```python
from build123d import *

# Parameters (mm, degrees)
SKETCH2_W                  = 68
SKETCH2_H                  = 65
BOSS_EXTRUDE1_DEPTH        = 3
SKETCH3_W                  = 3
SKETCH3_H                  = 65
BOSS_EXTRUDE2_DEPTH        = 62
CUT_EXTRUDE1_DEPTH         = 78.821912081
SKETCH5_R                  = 19.05
CUT_EXTRUDE2_DEPTH         = 100.525122457
F_5_5_5_5_DIAMETER_HOLE1_D = 5.5
CHAMFER1_SIZE              = 5
CHAMFER2_SIZE              = 5
CHAMFER3_SIZE              = 5
BOSS_EXTRUDE3_DEPTH        = 2.5
BOSS_EXTRUDE4_DEPTH        = 2.5


with BuildPart() as part:
    # Sketch2 → Boss-Extrude1 (new body)
    with BuildSketch(Plane(origin=(0, 0, 0), x_dir=(1, 0, 0), z_dir=(0, 1, 0))):
        Rectangle(SKETCH2_W, SKETCH2_H)
    extrude(amount=BOSS_EXTRUDE1_DEPTH)

    # Sketch3 → Boss-Extrude2 (add)
    with BuildSketch(Plane(origin=(0, 3, 0), x_dir=(1, 0, 0), z_dir=(0, 1, 0))):
        with Locations((-32.5, 0)):
            Rectangle(SKETCH3_W, SKETCH3_H)
    extrude(amount=BOSS_EXTRUDE2_DEPTH)

    # Sketch4 → Cut-Extrude1 (cut, through all)
    with BuildSketch(Plane(origin=(0, 3, 0), x_dir=(1, 0, 0), z_dir=(0, 1, 0))):
        with BuildLine():
            Line((-17.9, 22.5), (23.8, 22.5))
            ThreePointArc((23.8, 22.5), (26.3, 20), (23.8, 17.5))
            Line((23.8, 17.5), (-17.9, 17.5))
            ThreePointArc((-17.9, 17.5), (-20.4, 20), (-17.9, 22.5))
        make_face()
        with BuildLine():
            Line((-17.9, -17.5), (23.8, -17.5))
            ThreePointArc((23.8, -17.5), (26.3, -20), (23.8, -22.5))
            Line((23.8, -22.5), (-17.9, -22.5))
            ThreePointArc((-17.9, -22.5), (-20.4, -20), (-17.9, -17.5))
        make_face()
    extrude(amount=-CUT_EXTRUDE1_DEPTH, mode=Mode.SUBTRACT)

    # Sketch5 → Cut-Extrude2 (cut, through all)
    with BuildSketch(Plane.ZY.offset(34)):
        with Locations((0, 36)):
            Circle(SKETCH5_R)
    extrude(amount=-CUT_EXTRUDE2_DEPTH, mode=Mode.SUBTRACT)

    # Ø5.5 (5.5) Diameter Hole1 (through all)
    with Locations(Plane.ZY.offset(34)):
        with Locations((23.55, 59.55), (-23.55, 59.55), (-23.55, 12.45), (23.55, 12.45)):
            Hole(F_5_5_5_5_DIAMETER_HOLE1_D / 2)

    # Chamfer1
    chamfer1_edges = [part.edges().sort_by_distance(p)[0] for p in [
        (-32.5, 65, -32.5),
    ]]
    chamfer(chamfer1_edges, length=CHAMFER1_SIZE)

    # Chamfer2
    chamfer2_edges = [part.edges().sort_by_distance(p)[0] for p in [
        (-32.5, 65, 32.5),
    ]]
    chamfer(chamfer2_edges, length=CHAMFER2_SIZE)

    # Chamfer3
    chamfer3_edges = [part.edges().sort_by_distance(p)[0] for p in [
        (34, 1.5, 32.5),
        (34, 1.5, -32.5),
    ]]
    chamfer(chamfer3_edges, length=CHAMFER3_SIZE)

    # Sketch8 → Boss-Extrude3 (add)
    with BuildSketch(Plane.XY.offset(32.5)):
        Polygon((-31, 3), (-31, 28), (-11, 3), align=None)
    extrude(amount=-BOSS_EXTRUDE3_DEPTH)

    # Sketch9 → Boss-Extrude4 (add)
    with BuildSketch(Plane(origin=(0, 0, -32.5), x_dir=(-1, 0, 0), z_dir=(0, 0, -1))):
        Polygon((31, 3), (31, 28), (11, 3), align=None)
    extrude(amount=-BOSS_EXTRUDE4_DEPTH)


solid = part.part
```
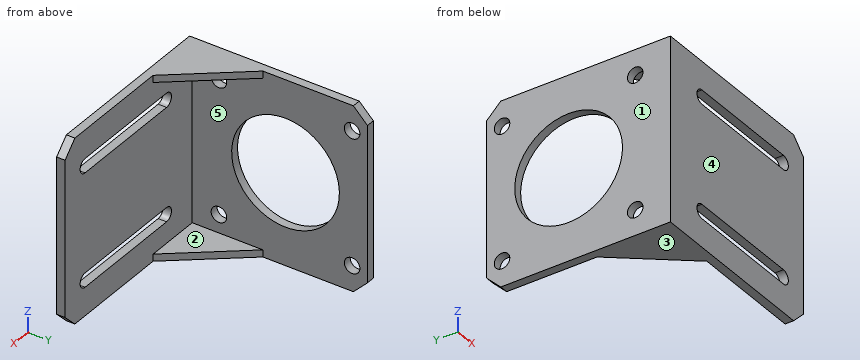
Build history of the part. All positions in model axes, mm. Face numbers are marked on the shaded views. A direction names the side the tool comes from. Coordinates: 2 decimals unless noted, no trailing zeros. Order: outer loops, then holes, each group sorted by start corner. A loop starts at its lowest first (then second) coordinate and runs counter-clockwise, first axis right, second up. Notation, with made-up numbers: (-36.75, 29) -> (-28.75, 29) arc R20 cw to (-28.75, 42) -> close; hole circle Ø8 at (-11.75, 11). An arc over 180 degrees is marked (long way). Answer in a Markdown table with one row per item. Add a question column.
Q1. Drop flat-ended pins along their axis: pin 1 (6 mm diameter, centred on y = 53.5, z = -11, fed in from +X); pin 2 (8 mm diameter, centred on x = 2, z = 10.5, fed in from +Y). Give the stop position or say it passes through.
Q2. Band-saw the part on A-A, the plane x = 4. List the corners of the cut face in (y, z), then the cut area to 3 significant figures.
Q3. Which spindle directions (+Z, -Z, +X, -X, +Y, -Y) get a long thin tool onto all of the face, cutting with end or side? Do the marked faces 4 and 5. Say none if no direction does.
Q4. Band-saw the part on D-D, the plane y = 12.45. List the corners of the cut face in (x, z).
Q5. Mould opens along Z. For the marked faces 1, 2 and 3 say: +Z half, -Z half, draft (parallel to the pull), parting line (faces both ways), or undercut.
Q6. Wall check: line 1 along Y through (x, z) = (-32.65, -23.55); line 2 along Y through (x, z) = (-32.95, 0); line 3 along X through (y, z) = (5, 3). Give the ranges that are in metal, low to high. Write a range as [from, to].
Q7. Band-saw the part on C-C, the plane z = -23.55. List the corners of the cut face in (x, y).
Q8. Band-saw the part on B-B, the plane y = 36. List the corners of the cut face in (x, z), then the cut area to 3 significant figures.
Answers follow:
| question | item | result |
|---|---|---|
| 1 | pin 1 | x = -31 |
| 1 | pin 2 | y = 3 |
| 2 | outline | (0, -32.5) -> (3, -32.5) -> (3, -22.5) -> (0, -22.5) -> close; (0, -17.5) -> (3, -17.5) -> (3, 17.5) -> (0, 17.5) -> close; (0, 22.5) -> (3, 22.5) -> (3, 32.5) -> (0, 32.5) -> close |
| 2 | area | 165 mm^2 |
| 3 | face 4 | +Z, -Z, +X, -X, -Y |
| 3 | face 5 | +X, +Y |
| 4 | outline | (-34, -32.5) -> (-18.56, -32.5) -> (-18.56, -30) -> (-31, -30) -> (-31, -26.3) -> (-34, -26.3) -> close; (-34, -20.8) -> (-31, -20.8) -> (-31, 20.8) -> (-34, 20.8) -> close; (-34, 26.3) -> (-31, 26.3) -> (-31, 30) -> (-18.56, 30) -> (-18.56, 32.5) -> (-34, 32.5) -> close |
| 5 | face 1 | draft |
| 5 | face 2 | undercut |
| 5 | face 3 | -Z half |
| 6 | line 1 | [0, 9.7], [15.2, 56.8], [62.3, 65] |
| 6 | line 2 | [0, 16.95], [55.05, 65] |
| 6 | line 3 | [-34, -31] |
| 7 | outline | (-34, 0) -> (34, 0) -> (34, 3) -> (-31, 3) -> (-31, 9.7) -> (-34, 9.7) -> close; (-34, 15.2) -> (-31, 15.2) -> (-31, 56.8) -> (-34, 56.8) -> close; (-34, 62.3) -> (-31, 62.3) -> (-31, 65) -> (-34, 65) -> close |
| 8 | outline | (-34, -32.5) -> (-31, -32.5) -> (-31, -19.05) -> (-34, -19.05) -> close; (-34, 19.05) -> (-31, 19.05) -> (-31, 32.5) -> (-34, 32.5) -> close |
| 8 | area | 80.7 mm^2 |
